Model file for the job. Use its own axes, mm. Face numbers are marked on the shaded views. A direction names the side the tool comes from. Coordinates: 2 decimals unless noted, no trailing zeros. Order: outer loops, then holes, each group sorted by start corner. A loop starts at its lowest first (then second) coordinate and runs counter-clockwise, first axis right, second up. Notation, with made-up numbers: (66.25, -8) -> (81.25, -8) arc R15 cw to (81.25, 3) -> close; hole circle Ø10 at (89, 17). An arc over 180 degrees is marked (long way). Return JSON: item names as keys, results as strings. Group by question number.
1) Cut at B-B (z = -32.14). State how many separate pieces and enclosed holes the cut face has, and give its area (3 significant figures).
2) Flat gauge pins, fed straight in: pin 1 (1.6 mm diameter, centred on x = 39.5, y = 9.5, fed in from -Z) (3 decimals); pin 2 (6 mm diameter, centred on x = 19, y = 23.5, fed in from -Z); pin 3 (1.3 mm diameter, centred on y = 3.09, z = -2.11, fed in from +X); pin 4 (1.6 mm diameter, centred on x = 40.5, y = 9, fed in from +Z) (3 decimals). Where does each tip first touch, or does it go through?
3) Which spindle directions (+Z, -Z, +X, -X, +Y, -Y) get a long thin tool onto all of the face, cutting with end or side? Do the marked faces 1, 2, 3 and 4. Say none if no direction does.
4) Probe line 1 (Z direction, x = 26, y = 13.5) (3 decimals); line 2 (Z direction, x = 20.79, y = 13.25) (3 decimals); line 3 (Y direction, x = 2, z = -2) (3 decimals). List the from-to ranges inside material, lowest first.
5) Cut at D-D (z = -4). Write the cut outline in (x, y) (3 decimals), and give its area (3 significant figures).
6) Pull direction Y, two halves, no side cores. Call the marked faces 5, 6 and 7: +Y half, -Y half, draft (parallel to the pull), parting line (faces both ways), or undercut.
from build123d import *

# Parameters (mm, degrees)
SKETCH1_W                       = 25
SKETCH1_H                       = 30
BOSS_EXTRUDE1_DEPTH             = 3.175
SKETCH2_W                       = 25
SKETCH2_H                       = 3.175
BOSS_EXTRUDE2_DEPTH             = 41.58
SKETCH3_W                       = 3.175
SKETCH3_H                       = 25
BOSS_EXTRUDE3_DEPTH             = 30
CUT_EXTRUDE1_REACH              = 60.775
SKETCH4_R                       = 11.5
CUT_EXTRUDE2_REACH              = 60.775
SKETCH5_R                       = 0.8
CUT_EXTRUDE3_REACH              = 60.775
SKETCH6_R                       = 0.8
SKETCH6_R_2                     = 0.799851166
SKETCH6_W                       = 21.2
SKETCH6_H                       = 6.375
CUT_EXTRUDE4_REACH              = 60.775
SKETCH7_R                       = 11.5
BOSS_EXTRUDE4_DEPTH             = 0.2
SKETCH9_W                       = 41.58
SKETCH9_H                       = 33.175
BOSS_EXTRUDE5_DEPTH             = 3.175
BOSS_EXTRUDE6_DEPTH             = 0.2
SKETCH11_W                      = 41.58
SKETCH11_H                      = 33.175
BOSS_EXTRUDE7_DEPTH             = 3.175
CHAMFER1_SIZE                   = 3.175
CHAMFER2_SIZE                   = 3.175
SKETCH13_W                      = 29.58
SKETCH13_H                      = 3.175
BOSS_EXTRUDE8_DEPTH             = 6.59
BOSS_EXTRUDE9_REACH             = 59.287
SKETCH14_W                      = 29.58
SKETCH14_H                      = 3.5
BOSS_EXTRUDE9_DIRECTION_2_DEPTH = 25
CHAMFER3_SIZE                   = 3.5
FILLET1_R                       = 1.5875
FILLET2_R                       = 1.5875
CUT_EXTRUDE5_REACH              = 69.476
SKETCH16_R                      = 4.6
SKETCH20_R                      = 8
SKETCH20_R_2                    = 2.6
BOSS_EXTRUDE11_DEPTH            = 5
CUT_EXTRUDE6_START              = -21.7275
SKETCH21_R                      = 1.025
CUT_EXTRUDE6_DEPTH              = 16
BOSS_EXTRUDE12_DEPTH            = 5
BOSS_EXTRUDE12_DEPTH_BACK       = 1.2
SKETCH23_R                      = 5.1
SKETCH23_R_2                    = 2.6


with BuildPart() as part:
    # Sketch1 → Boss-Extrude1 (new body)
    with BuildSketch(Plane(origin=(0, 0, 0), x_dir=(0, 0, -1), z_dir=(1, 0, 0))):
        with Locations((12.5, 15)):
            Rectangle(SKETCH1_W, SKETCH1_H)
    extrude(amount=BOSS_EXTRUDE1_DEPTH)

    # Sketch2 → Boss-Extrude2 (add)
    with BuildSketch(Plane.ZY):
        with Locations((-12.5, 31.5875)):
            Rectangle(SKETCH2_W, SKETCH2_H)
    extrude(amount=-BOSS_EXTRUDE2_DEPTH)

    # Sketch3 → Boss-Extrude3 (add)
    with BuildSketch(Plane.XZ.offset(-30)):
        with Locations((39.9925, -12.5)):
            Rectangle(SKETCH3_W, SKETCH3_H)
    extrude(amount=BOSS_EXTRUDE3_DEPTH)

    # Sketch4 → Cut-Extrude1 (cut, up to next)
    with BuildSketch(Plane.ZY, mode=Mode.PRIVATE) as cut_extrude1_sk1:
        with Locations((-12.359999929, -5.209996254)):
            Circle(SKETCH4_R)
    cut_extrude1_tool1 = extrude(cut_extrude1_sk1.sketch, amount=-CUT_EXTRUDE1_REACH, mode=Mode.PRIVATE) & part.part
    add(cut_extrude1_tool1.solids().sort_by_distance((0, -5.209996, -12.36))[0], mode=Mode.SUBTRACT)

    # Sketch5 → Cut-Extrude2 (cut, up to next)
    with BuildSketch(Plane.ZY, mode=Mode.PRIVATE) as cut_extrude2_sk1:
        with Locations((-22.609999929, 3.090003746)):
            Circle(SKETCH5_R)
    cut_extrude2_tool1 = extrude(cut_extrude2_sk1.sketch, amount=-CUT_EXTRUDE2_REACH, mode=Mode.PRIVATE) & part.part
    # Sketch5 → Cut-Extrude2 (cut, up to next)
    with BuildSketch(Plane.ZY, mode=Mode.PRIVATE) as cut_extrude2_sk2:
        with Locations((-22.609999929, 23.790003746)):
            Circle(SKETCH5_R)
    cut_extrude2_tool2 = extrude(cut_extrude2_sk2.sketch, amount=-CUT_EXTRUDE2_REACH, mode=Mode.PRIVATE) & part.part
    # Sketch5 → Cut-Extrude2 (cut, up to next)
    with BuildSketch(Plane.ZY, mode=Mode.PRIVATE) as cut_extrude2_sk3:
        with Locations((-2.109999929, 23.790003746)):
            Circle(SKETCH5_R)
    cut_extrude2_tool3 = extrude(cut_extrude2_sk3.sketch, amount=-CUT_EXTRUDE2_REACH, mode=Mode.PRIVATE) & part.part
    # Sketch5 → Cut-Extrude2 (cut, up to next)
    with BuildSketch(Plane.ZY, mode=Mode.PRIVATE) as cut_extrude2_sk4:
        with Locations((-2.109999929, 3.090003746)):
            Circle(SKETCH5_R)
    cut_extrude2_tool4 = extrude(cut_extrude2_sk4.sketch, amount=-CUT_EXTRUDE2_REACH, mode=Mode.PRIVATE) & part.part
    add(cut_extrude2_tool1.solids().sort_by_distance((0, 3.090004, -22.61))[0], mode=Mode.SUBTRACT)
    add(cut_extrude2_tool2.solids().sort_by_distance((0, 23.790004, -22.61))[0], mode=Mode.SUBTRACT)
    add(cut_extrude2_tool3.solids().sort_by_distance((0, 23.790004, -2.11))[0], mode=Mode.SUBTRACT)
    add(cut_extrude2_tool4.solids().sort_by_distance((0, 3.090004, -2.11))[0], mode=Mode.SUBTRACT)

    # Sketch6 → Cut-Extrude3 (cut, up to next)
    with BuildSketch(Plane(origin=(41.58, 0, 0), x_dir=(0, 0, -1), z_dir=(1, 0, 0)), mode=Mode.PRIVATE) as cut_extrude3_sk1:
        with Locations(Location((2.109999929, 3.090003746, 0), (0, 0, 180))):
            Circle(SKETCH6_R)
    cut_extrude3_tool1 = extrude(cut_extrude3_sk1.sketch, amount=-CUT_EXTRUDE3_REACH, mode=Mode.PRIVATE) & part.part
    # Sketch6 → Cut-Extrude3 (cut, up to next)
    with BuildSketch(Plane(origin=(41.58, 0, 0), x_dir=(0, 0, -1), z_dir=(1, 0, 0)), mode=Mode.PRIVATE) as cut_extrude3_sk2:
        with Locations(Location((22.609999929, 3.090003746, 0), (0, 0, 180))):
            Circle(SKETCH6_R)
    cut_extrude3_tool2 = extrude(cut_extrude3_sk2.sketch, amount=-CUT_EXTRUDE3_REACH, mode=Mode.PRIVATE) & part.part
    # Sketch6 → Cut-Extrude3 (cut, up to next)
    with BuildSketch(Plane(origin=(41.58, 0, 0), x_dir=(0, 0, -1), z_dir=(1, 0, 0)), mode=Mode.PRIVATE) as cut_extrude3_sk3:
        with Locations((22.609999929, 27.540003746)):
            Circle(SKETCH6_R_2)
    cut_extrude3_tool3 = extrude(cut_extrude3_sk3.sketch, amount=-CUT_EXTRUDE3_REACH, mode=Mode.PRIVATE) & part.part
    # Sketch6 → Cut-Extrude3 (cut, up to next)
    with BuildSketch(Plane(origin=(41.58, 0, 0), x_dir=(0, 0, -1), z_dir=(1, 0, 0)), mode=Mode.PRIVATE) as cut_extrude3_sk4:
        with Locations((2.109999929, 27.540003746)):
            Circle(SKETCH6_R)
    cut_extrude3_tool4 = extrude(cut_extrude3_sk4.sketch, amount=-CUT_EXTRUDE3_REACH, mode=Mode.PRIVATE) & part.part
    # Sketch6 → Cut-Extrude3 (cut, up to next)
    with BuildSketch(Plane(origin=(41.58, 0, 0), x_dir=(0, 0, -1), z_dir=(1, 0, 0)), mode=Mode.PRIVATE) as cut_extrude3_sk5:
        with Locations((12.359999929, 8.927503746)):
            Rectangle(SKETCH6_W, SKETCH6_H)
    cut_extrude3_tool5 = extrude(cut_extrude3_sk5.sketch, amount=-CUT_EXTRUDE3_REACH, mode=Mode.PRIVATE) & part.part
    add(cut_extrude3_tool1.solids().sort_by_distance((41.58, 3.090004, -2.11))[0], mode=Mode.SUBTRACT)
    add(cut_extrude3_tool2.solids().sort_by_distance((41.58, 3.090004, -22.61))[0], mode=Mode.SUBTRACT)
    add(cut_extrude3_tool3.solids().sort_by_distance((41.58, 27.540004, -22.61))[0], mode=Mode.SUBTRACT)
    add(cut_extrude3_tool4.solids().sort_by_distance((41.58, 27.540004, -2.11))[0], mode=Mode.SUBTRACT)
    add(cut_extrude3_tool5.solids().sort_by_distance((41.58, 8.927504, -12.36))[0], mode=Mode.SUBTRACT)

    # Sketch7 → Cut-Extrude4 (cut, up to next)
    with BuildSketch(Plane(origin=(41.58, 0, 0), x_dir=(0, 0, -1), z_dir=(1, 0, 0)), mode=Mode.PRIVATE) as cut_extrude4_sk1:
        with Locations((12.359999929, -5.209996254)):
            Circle(SKETCH7_R)
    cut_extrude4_tool1 = extrude(cut_extrude4_sk1.sketch, amount=-CUT_EXTRUDE4_REACH, mode=Mode.PRIVATE) & part.part
    add(cut_extrude4_tool1.solids().sort_by_distance((41.58, -5.209996, -12.36))[0], mode=Mode.SUBTRACT)

    # Sketch8 → Boss-Extrude4 (add)
    with BuildSketch(Plane.XY):
        Polygon((0, 33.175), (0, 0), (3.175, 0), (3.175, 30), (38.405, 30), (38.405, 0), (41.58, 0), (41.58, 33.175), align=None)
    extrude(amount=BOSS_EXTRUDE4_DEPTH)

    # Sketch9 → Boss-Extrude5 (add)
    with BuildSketch(Plane.XY.offset(0.2)):
        with Locations((20.79, 16.5875)):
            Rectangle(SKETCH9_W, SKETCH9_H)
    extrude(amount=BOSS_EXTRUDE5_DEPTH)

    # Sketch10 → Boss-Extrude6 (add)
    with BuildSketch(Plane(origin=(0, 0, -25), x_dir=(-1, 0, 0), z_dir=(0, 0, -1))):
        Polygon((0, 0), (0, 33.175), (-41.58, 33.175), (-41.58, 0), (-38.405, 0), (-38.405, 30), (-3.175, 30), (-3.175, 0), align=None)
    extrude(amount=BOSS_EXTRUDE6_DEPTH)

    # Sketch11 → Boss-Extrude7 (add)
    with BuildSketch(Plane(origin=(0, 0, -25.2), x_dir=(-1, 0, 0), z_dir=(0, 0, -1))):
        with Locations((-20.79, 16.5875)):
            Rectangle(SKETCH11_W, SKETCH11_H)
    extrude(amount=BOSS_EXTRUDE7_DEPTH)

    # Chamfer1
    chamfer1_edges = [part.edges().sort_by_distance(p)[0] for p in [
        (20.79, 33.175, 3.375),
        (20.79, 33.175, -28.375),
    ]]
    chamfer(chamfer1_edges, length=CHAMFER1_SIZE)

    # Chamfer2
    chamfer2_edges = [part.edges().sort_by_distance(p)[0] for p in [
        (20.79, 0, 3.375),
        (20.79, 0, -28.375),
    ]]
    chamfer(chamfer2_edges, length=CHAMFER2_SIZE - 0.0001)  # a hair under: the kernel refuses the full size

    # Sketch13 → Boss-Extrude8 (add)
    with BuildSketch(Plane(origin=(0, 0, -28.375), x_dir=(-1, 0, 0), z_dir=(0, 0, -1))):
        with Locations((-20.79, 19.7625)):
            Rectangle(SKETCH13_W, SKETCH13_H)
    extrude(amount=BOSS_EXTRUDE8_DEPTH)

    # Boss-Extrude9: up to this face of the body (flat: up to its plane)
    boss_extrude9_end = Plane(part.part.faces().sort_by_distance((20.79, 21.35, -31.67))[0])
    # Sketch14 → Boss-Extrude9 (add, up to the picked face)
    with BuildSketch(Plane.XZ.offset(-18.175), mode=Mode.PRIVATE) as boss_extrude9_sk1:
        with Locations((20.79, -36.39)):
            Rectangle(SKETCH14_W, SKETCH14_H)
    boss_extrude9_tool1 = split(extrude(boss_extrude9_sk1.sketch, amount=-BOSS_EXTRUDE9_REACH, mode=Mode.PRIVATE), bisect_by=boss_extrude9_end, keep=Keep.BOTH, mode=Mode.PRIVATE)
    add(boss_extrude9_tool1.solids().sort_by(Axis((20.79, 18.175, -36.39), (0, 1, 0)))[0])

    # Sketch14 → Boss-Extrude9 direction 2 (add)
    with BuildSketch(Plane.XZ.offset(-18.175)):
        with Locations((20.79, -36.39)):
            Rectangle(SKETCH14_W, SKETCH14_H)
    extrude(amount=BOSS_EXTRUDE9_DIRECTION_2_DEPTH)

    # Chamfer3
    chamfer3_edges = [part.edges().sort_by_distance(p)[0] for p in [
        (6, -6.825, -36.39),
        (35.58, -6.825, -36.39),
    ]]
    chamfer(chamfer3_edges, length=CHAMFER3_SIZE)

    # Fillet1
    fillet1_edges = [part.edges().sort_by_distance(p)[0] for p in [
        (20.79, 18.175, -34.64),
        (20.79, 21.35, -38.14),
    ]]
    fillet(fillet1_edges, radius=FILLET1_R)

    # Fillet2
    fillet2_edges = [part.edges().sort_by_distance(p)[0] for p in [
        (20.79, 21.35, -28.375),
    ]]
    fillet(fillet2_edges, radius=FILLET2_R)

    # Sketch16 → Cut-Extrude5 (cut, up to next)
    with BuildSketch(Plane(origin=(0, 0, -38.14), x_dir=(-1, 0, 0), z_dir=(0, 0, -1)), mode=Mode.PRIVATE) as cut_extrude5_sk1:
        with Locations((-20.79, 6.9025)):
            Circle(SKETCH16_R)
    cut_extrude5_tool1 = extrude(cut_extrude5_sk1.sketch, amount=-CUT_EXTRUDE5_REACH, mode=Mode.PRIVATE) & part.part
    add(cut_extrude5_tool1.solids().sort_by_distance((20.79, 6.9025, -38.14))[0], mode=Mode.SUBTRACT)

    # Sketch20 → Boss-Extrude11 (add)
    with BuildSketch(Plane.XY.offset(-34.64)):
        with Locations(Location((20.79, 6.9025, 0), (0, 0, 180))):
            Circle(SKETCH20_R)
        with Locations((20.79, 6.9025)):
            Circle(SKETCH20_R_2, mode=Mode.SUBTRACT)
    extrude(amount=BOSS_EXTRUDE11_DEPTH)

    # Sketch21 → Cut-Extrude6 (cut)
    with BuildSketch(Plane.XZ.offset(6.825).offset(CUT_EXTRUDE6_START)):
        with Locations(Location((20.79, -32.14, 0), (0, 0, 270))):
            Circle(SKETCH21_R)
    extrude(amount=CUT_EXTRUDE6_DEPTH, mode=Mode.SUBTRACT)

    # Sketch23 → Boss-Extrude12 (add, two sides: drawn at the far end of the back side and taken through both)
    with BuildSketch(Plane.XY.offset(3.375).offset(-BOSS_EXTRUDE12_DEPTH_BACK)):
        with Locations(Location((20.79, 6.9025, 0), (0, 0, 226.960415899))):
            Circle(SKETCH23_R)
        with Locations((20.79, 6.9025)):
            Circle(SKETCH23_R_2, mode=Mode.SUBTRACT)
    extrude(amount=BOSS_EXTRUDE12_DEPTH + BOSS_EXTRUDE12_DEPTH_BACK)


solid = part.part
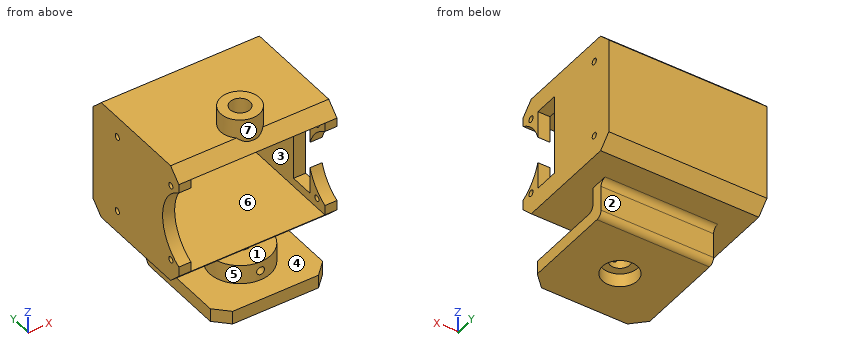
Answers below:
{
 "1": {"separate pieces": "3", "enclosed holes": "0", "area": "251 mm^2"},
 "2": {"pin 1": "stops at z = -28.375", "pin 2": "stops at z = -37.96", "pin 3": "passes through", "pin 4": "stops at z = 3.375"},
 "3": {"face 1": "+X, -X, -Y", "face 2": "-Z, +X, -X, +Y", "face 3": "-Y", "face 4": "none"},
 "4": {"line 1": "z = -38.14 to -34.64, -28.375 to -25.2, 0.2 to 3.375", "line 2": "z = -38.14 to -33.165, -31.115 to -29.64, -28.375 to -25.2, 0.2 to 3.375", "line 3": "y = 0 to 2.298, 3.882 to 22.998, 24.582 to 33.175"},
 "5": {"outline": "(0, 2.687) -> (3.175, 2.687) -> (3.175, 30) -> (38.405, 30) -> (38.405, 12.115) -> (41.58, 12.115) -> (41.58, 33.175) -> (0, 33.175) -> close; (38.405, 2.687) -> (41.58, 2.687) -> (41.58, 5.74) -> (38.405, 5.74) -> close", "area": "285 mm^2"},
 "6": {"face 5": "undercut", "face 6": "draft", "face 7": "parting line"}
}
